The listing builds one solid part. Answer for the finished solid, in the listing's coordinates (mm). Coordinates: 2 decimals unless noted, no trailing zeros. Write each loop counter-clockwise with the first axis right and the second up, starting at its lowest first coordinate (ties: lowest second). Pieces come first, ordered by that corner, then holes.
from build123d import *

# Parameters (mm, degrees)
SKETCH10_R          = 30
SKETCH10_R_2        = 9.875
BOSS_EXTRUDE4_DEPTH = 10
FILLET1_R           = 4
FILLET2_R           = 5


with BuildPart() as part:
    # Sketch10 → Boss-Extrude4 (new body)
    with BuildSketch(Plane.XY):
        with Locations((-81.433006588, 0)):
            Circle(SKETCH10_R)
        with Locations((-81.433006588, 0)):
            Circle(SKETCH10_R_2, mode=Mode.SUBTRACT)
    extrude(amount=BOSS_EXTRUDE4_DEPTH)

    # Fillet1
    fillet1_edges = [part.edges().sort_by_distance(p)[0] for p in [
        (-111.433006588, 0, 10),
    ]]
    fillet(fillet1_edges, radius=FILLET1_R)

    # Fillet2
    fillet2_edges = [part.edges().sort_by_distance(p)[0] for p in [
        (-91.308006588, 0, 0),
    ]]
    fillet(fillet2_edges, radius=FILLET2_R)


solid = part.part
Q1. Find the intervals of material crossed by probe 1 along X at (y, z) = (-2.5, 2.75); probe 2 along X at (y, z) = (-7, 5.75); probe 3 along Y at (x, z) = (-70.5, 2), in increasing order.
Answers below:
probe 1: x = -111.33 to -91.54, -71.33 to -51.54
probe 2: x = -110.6 to -88.4, -74.47 to -52.26
probe 3: y = -27.94 to 27.94
Q2. The part is cut by section C-C, the plane z = 8.25. Write down the section's boundary in (x, y) (3 decimals), then the cut area to 3 significant figures.
Answers below:
outline: circle Ø58.614 at (-81.433, 0); hole circle Ø19.75 at (-81.433, 0)
area: 2,390 mm2
Q3. Determine the mould class of faces 1 (the face through (-75, 14, 0)), 2 (the face through (-91.3, 0.4, 7.5)), 3 (the face through (-111.404, 1.319, 2.958)) for opening direction Y: released by +Y, released by -Y, zero draft, split by the parting line, or undercut.
Answers below:
face 1: zero draft
face 2: undercut
face 3: split by the parting line
Q4. The part is cut by section B-B, the plane z = 4.25. Write down the section's boundary in (x, y), then the cut area to 3 significant figures.
Answers below:
outline: circle Ø60 at (-81.43, 0); hole circle Ø19.86 at (-81.43, 0)
area: 2,520 mm2
Q5. The part is cut by section A-A, the plane y = 0. Write down the section's boundary in (x, z).
Answers below:
outline: (-111.43, 0) - (-96.31, 0) arc R5 ccw to (-91.31, 5) - (-91.31, 10) - (-107.43, 10) arc R4 ccw to (-111.43, 6) - close; (-71.56, 5) arc R5 ccw to (-66.56, 0) - (-51.43, 0) - (-51.43, 6) arc R4 ccw to (-55.43, 10) - (-71.56, 10) - close
Q6. Given pin 1 (12 mm diameter, centred on x = -81.43, y = 0, fed in from +Z); pin 2 (3 mm diameter, centred on x = -94, z = 2.5, fed in from +Y); pin 3 (5 mm diameter, centred on x = -95, z = 9, fed in from -Y); pin 4 (5 mm diameter, centred on x = -75, z = 7.5, fed in from -Y), each flat-ended and moving along its own axis, determine where each tip first touches the part or whether it passes through.
Answers below:
pin 1: passes through
pin 2: stops at y = 27.88
pin 3: stops at y = -27.37
pin 4: stops at y = -29.69
